from build123d import *

# Parameters (mm, degrees)
EXTRUDE_1_DEPTH     = 8.75
CUT_EXTRUDE_1_REACH = 20.251
SKETCH_3_R          = 2


with BuildPart() as part:
    # 草圖1 → 填料-伸長1 (new, symmetric)
    with BuildSketch(Plane(origin=(0, 0, 0), x_dir=(0, 0, -1), z_dir=(1, 0, 0))):
        with BuildLine():
            Line((-3.250001327, 2.120345625), (3.250001327, 2.120345625))
            ThreePointArc((3.250001327, 2.120345625), (5.267515394, -0.02636871), (6.00066364, -2.879654375))
            Line((6.00066364, -2.879654375), (15, -2.879654375))
            Line((15, -2.879654375), (15, -0.382935225))
            Line((15, -0.382935225), (8, -0.382935225))
            Line((8, -0.382935225), (8, 5.617064775))
            Line((8, 5.617064775), (-8, 5.617064775))
            Line((-8, 5.617064775), (-8, -0.382935225))
            Line((-8, -0.382935225), (-15, -0.382935225))
            Line((-15, -0.382935225), (-15, -2.879654375))
            Line((-15, -2.879654375), (-5.999788855, -2.879654375))
            ThreePointArc((-5.999788855, -2.879654375), (-5.267080125, -0.026479896), (-3.250001327, 2.120345625))
        make_face()
    extrude(amount=EXTRUDE_1_DEPTH, both=True)

    # 草圖3 → 除料-伸長1 (cut, up to next)
    with BuildSketch(Plane(origin=(0, 0, 0), x_dir=(1, 0, 0), z_dir=(0, 1, 0)), mode=Mode.PRIVATE) as cut_extrude_1_sk1:
        with Locations(Location((0, 11.5, 0), (0, 0, 270))):
            Circle(SKETCH_3_R)
    cut_extrude_1_tool1 = extrude(cut_extrude_1_sk1.sketch, amount=-CUT_EXTRUDE_1_REACH, mode=Mode.PRIVATE) & part.part
    # 草圖3 → 除料-伸長1 (cut, up to next)
    with BuildSketch(Plane(origin=(0, 0, 0), x_dir=(1, 0, 0), z_dir=(0, 1, 0)), mode=Mode.PRIVATE) as cut_extrude_1_sk2:
        with Locations(Location((0, -11.5, 0), (0, 0, 270))):
            Circle(SKETCH_3_R)
    cut_extrude_1_tool2 = extrude(cut_extrude_1_sk2.sketch, amount=-CUT_EXTRUDE_1_REACH, mode=Mode.PRIVATE) & part.part
    add(cut_extrude_1_tool1.solids().sort_by_distance((0, 0, -11.5))[0], mode=Mode.SUBTRACT)
    add(cut_extrude_1_tool2.solids().sort_by_distance((0, 0, 11.5))[0], mode=Mode.SUBTRACT)


solid = part.part
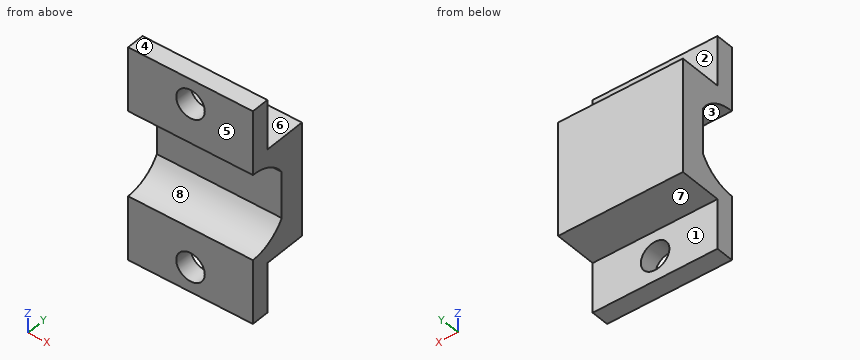
Could you check a few things on this model? Use its own coordinates, in mm. Face numbers are marked on the shaded views. A direction names the side the tool comes from. Give positions to 0.01 mm unless a question says otherwise; leave off trailing zeros. Order: outer loops, then holes, each group sorted by start corner. A loop starts at its lowest first (then second) coordinate and runs counter-clockwise, first axis right, second up. Notation, with made-up numbers: (33.25, -12) - (43.25, -12) arc R26 ccw to (43.25, 20) - close; hole circle Ø4 at (58, 77). An arc over 180 degrees is marked (long way). One line per question, with ' | ' between items. Start each with the question number.
Item 1: Thinking about a two-plate mould opening in Z: for the marked faces 5, 6, 7 and 8, which applies, pulls with the +Z half, pulls with the -Z half, needs draft (parallel to the pull), parting line crosses it, or undercut?
Item 2: I want a section at C-C on y = 0.25. Write out the boundary of the cut face in (x, z), then the cut area to 3 significant figures.
Item 3: For the marked faces 1, 2, 3 and 4, which set-ups out of +Z, -Z, +X, -X, +Y, -Y let a thin tool reach every point of the face, with its end or its side?
Item 4: I'm going to push flat-ended pins straight in: pin 1 Ø2 at (x, z) = (4, -12.5) entering from +Y; pin 2 Ø5 at (x, y) = (-4, 3.5) entering from -Z; pin 3 Ø2 at (x, z) = (1.5, -0.5) entering from -Y. Where does each tip first touch, or does it pass through?
Item 5: I need wall thicknesses on probe 1 along Y at (x, z) = (3.5, -9.75); probe 2 along X at (y, z) = (-1, 11.5); probe 3 along Y at (x, z) = (7.5, -0.25). Which ranges of each line are inside material? Lowest first, please. Write a range as [from, to].
Item 6: I want a section at B-B on x = 3. Write out the boundary of the cut face in (y, z), then the cut area to 3 significant figures.
Item 7: I want a section at D-D on z = 0.5. Write out the boundary of the cut face in (x, y), then the cut area to 3 significant figures.
Item 8: I want a section at A-A on z = -11.5. Write out the boundary of the cut face in (x, y).
Verdict:
1) face 5: needs draft | face 6: pulls with the +Z half | face 7: pulls with the -Z half | face 8: undercut
2) outline: (-8.75, -8) - (8.75, -8) - (8.75, -5.11) - (-8.75, -5.11) - close; (-8.75, 5.11) - (8.75, 5.11) - (8.75, 8) - (-8.75, 8) - close | area: 101 mm^2
3) face 1: -Z, +X, -X, +Y | face 2: +Z, +X, -X, +Y | face 3: +X, -X, -Y | face 4: +Z, +X, -X, +Y, -Y
4) pin 1: y = -0.38 | pin 2: z = -8 | pin 3: y = 2.12
5) probe 1: [-2.88, -0.38] | probe 2: [-8.75, -2], [2, 8.75] | probe 3: [2.12, 5.62]
6) outline: (-2.88, -15) - (-0.38, -15) - (-0.38, -8) - (5.62, -8) - (5.62, 8) - (-0.38, 8) - (-0.38, 15) - (-2.88, 15) - (-2.88, 6) arc R5.92 cw to (2.12, 3.25) - (2.12, -3.25) arc R5.92 cw to (-2.88, -6) - close | area: 119 mm^2
7) outline: (-8.75, 2.12) - (8.75, 2.12) - (8.75, 5.62) - (-8.75, 5.62) - close | area: 61.2 mm^2
8) outline: (-8.75, -2.88) - (-2, -2.88) - (-2, -0.38) - (-8.75, -0.38) - close; (2, -2.88) - (8.75, -2.88) - (8.75, -0.38) - (2, -0.38) - close
